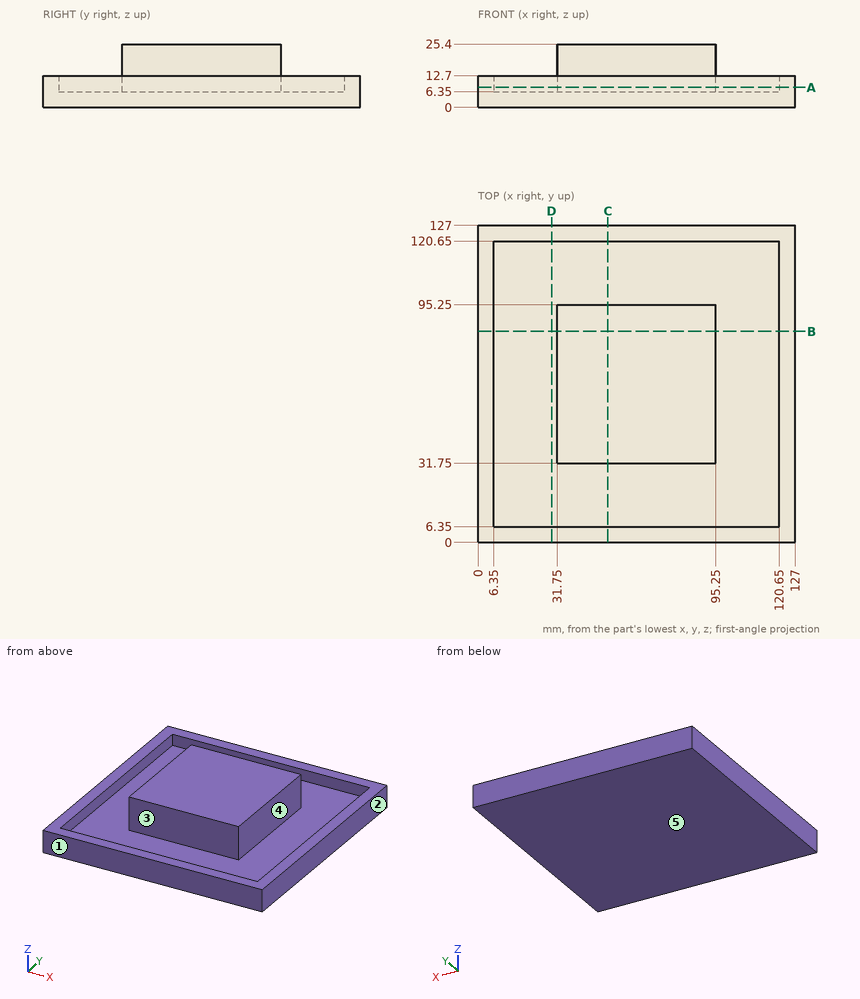
Geometry: see drawing. Coordinates: mm, zero at the bounding-box minimum. A direction names the side the tool comes from. Give positions to 0.01 mm unless a question says otherwise; leave off trailing zeros. Write each loop counter-clockwise with the first axis right and the second up, starting at its lowest first coordinate (ties: lowest second). Pieces come first, ordered by that corner, then holes. Notation, with made-up numbers: M -28,44.25 L -24,44.25 A6 ccw -24,48.25 Z; hole C 31,-19 d6. An arc over 180 degrees is marked long. Answer in a Markdown table with one row per item. Add a question column.
(1) Section A-A on z = 8. Return loops of the section in (x, y), and give its area (3 significant figures).
(2) Section D-D on x = 29.5. Return loops of the section in (y, z).
(3) Section B-B on y = 84.5. Return loops of the section in (x, z).
(4) Ray query, line 1 (X direction, y = 92.5, z = 7.75); line 2 (X direction, y = 117, z = 7.5). Return the intervals inside material, ascending.
(5) Reachability of the marked faces 4 and 5 from +Z, -Z, +X, -X, +Y, -Y: full face, straight path, thin tool, end or side. Return the list, or none.
(6) First-contact query: pin 1 (5.5 mm diameter, centred on x = 62, z = 15.5, fed in from +Y); pin 2 (8 mm diameter, centred on y = 86.5, z = 17, fed in from +X). Flat tips, straight axial feed; report the tip coordinate or a pass-through.
(7) Mould query, pull axis X, two halves, no side actions, for the marked faces 1, 2 and 3. Classes: +X half, -X half, draft (parallel to the pull), parting line (faces both ways), or undercut.
Result set:
| question | item | result |
|---|---|---|
| 1 | outline | M 0,0 L 127,0 L 127,127 L 0,127 Z; M 31.75,31.75 L 95.25,31.75 L 95.25,95.25 L 31.75,95.25 Z; hole M 6.35,6.35 L 120.65,6.35 L 120.65,120.65 L 6.35,120.65 Z |
| 1 | area | 7,100 mm^2 |
| 2 | outline | M 0,0 L 127,0 L 127,12.7 L 120.65,12.7 L 120.65,6.35 L 6.35,6.35 L 6.35,12.7 L 0,12.7 Z |
| 3 | outline | M 0,0 L 127,0 L 127,12.7 L 120.65,12.7 L 120.65,6.35 L 95.25,6.35 L 95.25,25.4 L 31.75,25.4 L 31.75,6.35 L 6.35,6.35 L 6.35,12.7 L 0,12.7 Z |
| 4 | line 1 | x = 0 to 6.35, 31.75 to 95.25, 120.65 to 127 |
| 4 | line 2 | x = 0 to 6.35, 120.65 to 127 |
| 5 | face 4 | +Z |
| 5 | face 5 | -Z, +X, -X, +Y, -Y |
| 6 | pin 1 | stops at y = 95.25 |
| 6 | pin 2 | stops at x = 95.25 |
| 7 | face 1 | draft |
| 7 | face 2 | +X half |
| 7 | face 3 | undercut |
